from build123d import *

# Parameters (mm, degrees)
F1_DEPTH    = 2
F2_R        = 1
F3_DEPTH    = 25
F4_R        = 1.15
F5_DEPTH    = 3
F6_T1_DEPTH = 2


# Not quite as in the source:
# - a fillet or chamfer that OpenCascade refuses, or shapes differently, is made with other operations: its cross-section is extruded or revolved along the edge and cut away or added


with BuildPart() as f1:
    # F0 (on Right) → F1 (new body)
    with BuildSketch(Plane.YZ):
        with BuildLine():
            Line((20, -8.475), (20, 8.475))
            Line((20, 8.475), (12.3, 8.475))
            Line((12.3, 8.475), (6.9, 0.475))
            Line((6.9, 0.475), (0, 0.475))
            Line((0, 0.475), (-6.9, 0.475))
            Line((-6.9, 0.475), (-12.3, 8.475))
            Line((-12.3, 8.475), (-20, 8.475))
            Line((-20, 8.475), (-20, -8.475))
            ThreePointArc((-20, -8.475), (0, -28.475), (20, -8.475))
        make_face()
    extrude(amount=F1_DEPTH)

    # F2 (on face) → F3 (cut)
    with BuildSketch(Plane.YZ.offset(2)):
        with Locations((0, -22.5554741919)):
            Circle(F2_R)
        with Locations((-12.6950368285, -14.3941175193)):
            Circle(F2_R)
        with Locations((-15.2600342408, 2.045188332)):
            Circle(F2_R)
        with Locations((12.6950368285, -14.3941175193)):
            Circle(F2_R)
        with Locations((15.2600342408, 2.045188332)):
            Circle(F2_R)
    extrude(amount=-F3_DEPTH, mode=Mode.SUBTRACT)

    # F4 (on face) → F5 (join)
    with BuildSketch(Plane(origin=(0, 20, 0), x_dir=(-1, 0, 0), z_dir=(0, 1, 0))):
        Polygon((0, 8.475), (0, 26.475), (-7.5, 26.475), (-7.5, 8.475), (-2, -8.475), (0, -8.475), align=None)
        with Locations((-3.75, 23.475)):
            Circle(F4_R, mode=Mode.SUBTRACT)
        Polygon((-2, -8.475), (-7.5, 8.475), (-7.5, -8.475), align=None)
    extrude(amount=F5_DEPTH)

    # F6: fillet of radius 5 on 1 edges, made by hand

    # F6_s2 → F6_t1 (join)
    with BuildSketch(Plane.YZ):
        with BuildLine():
            ThreePointArc((19.6347826087, -12.2796434668), (20.7982860057, -9.9181716989), (23, -8.475))
            Line((23, -8.475), (20, -8.475))
            ThreePointArc((20, -8.475), (19.9084862832, -10.3860661718), (19.6347826087, -12.2796434668))
        make_face()
    extrude(amount=F6_T1_DEPTH)


solid = f1.part
Read the model definition and answer for the solid it produces. Units are mm, in the model's axes. A direction names the side the tool comes from. Round coordinates to 2 decimals unless told otherwise and drop trailing zeros. Loops run counter-clockwise (first coordinate to the right, second up) from the corner with the lowest first, then second, coordinate; pieces in that order, holes last.
Q1. Which of the six approach directions +Z, -Z, +X, -X, +Y, -Y give full straight-line access (tool end or side, diameter ignored) to faces 1 (the face through (0.986, 9.638, 4.531)), 2 (the face through (1, 16, 8.475)), 3 (the face through (5, 21, -8.475)), 4 (the face through (1, -20, 0)), 5 (the face through (1.014, -11.771, -14.777))?
Q2. Determine the mould class of faces 6 (the face through (0.986, -9.562, 4.419)), 7 (the face through (0.99, 20.77, -9.95)), 8 (the face through (0.99, -2.32, -28.34)) for opening direction Y: released by +Y, released by -Y, zero draft, split by the parting line, or undercut.
Q3. Section A-A on x = 3.75 is taken. Write down the section's boundary in (y, z) (3 decimals).
Q4. Section D-D on z = 17 is taken. Write down the section's boundary in (x, y), and give its area (3 significant figures).
Q5. Each of these flat-tipped pins is pushed along its axis until it touches: pin 1 (1.8 mm diameter, centred on y = -12.7, z = -14.39, fed in from +X); pin 2 (2 mm diameter, centred on x = 1.5, y = 1, fed in from +Z) (3 decimals); pin 3 (1.5 mm diameter, centred on x = 1, y = 14, fed in from +Z) (3 decimals); pin 4 (4 mm diameter, centred on x = 2, z = 17.5, fed in from -Y). Where does it stop, or does it pass through?
Q6. Section C-C on z = -6 is taken. Write down the section's boundary in (x, y), and give its area (4 significant figures).
Q7. Section B-B on y = 0 is taken. Write down the section's boundary in (x, z) (3 decimals).
Q8. Consider probe 1 along Y at (x, z) = (4.5, 16); probe 2 along X at (y, z) = (-15.5, -12.5); probe 3 along Z at (x, y) = (1, -14.5) (3 decimals). Determine where each line is inside the solid, lowest interval first.
Output:
1. face 1: +Z, +X, -X
1. face 2: +Z, +X, -X, -Y
1. face 3: -Z, +X, +Y, -Y
1. face 4: +Z, -Z, +X, -X, -Y
1. face 5: +X, -X
2. face 6: undercut
2. face 7: released by +Y
2. face 8: split by the parting line
3. outline: (20, -8.475) - (23, -8.475) - (23, 22.325) - (20, 22.325) - close; (20, 24.625) - (23, 24.625) - (23, 26.475) - (20, 26.475) - close
4. outline: (0, 20) - (7.5, 20) - (7.5, 23) - (0, 23) - close
4. area: 22.5 mm2
5. pin 1: passes through
5. pin 2: stops at z = 0.475
5. pin 3: stops at z = 8.475
5. pin 4: stops at y = 20
6. outline: (0, -20) - (2, -20) - (2, 20) - (7.5, 20) - (7.5, 23) - (0, 23) - close
6. area: 102.5 mm2
7. outline: (0, -28.475) - (2, -28.475) - (2, -23.555) - (0, -23.555) - close; (0, -21.555) - (2, -21.555) - (2, 0.475) - (0, 0.475) - close
8. probe 1: y = 20 to 23
8. probe 2: x = 0 to 2
8. probe 3: z = -22.25 to 1.395, 2.695 to 8.475
